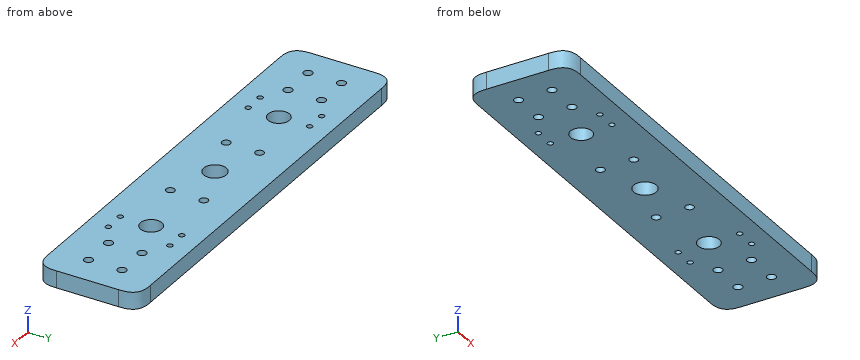
from build123d import *

# Parameters (mm, degrees)
SKETCH1_W                     = 320
SKETCH1_H                     = 76.2
BOSS_EXTRUDE1_DEPTH           = 12.7
M6_CLEARANCE_HOLE1_D          = 6.6
FILLET1_SIZE                  = 15
TAP_DRILL_FOR_M5X0_8_TAP1_D   = 4.2
SKETCH8_R                     = 8
CUT_EXTRUDE1_DEPTH            = 165.963329386
M6_CLEARANCE_HOLE2_D          = 6.4
M16_CLEARANCE_HOLE1_OUTLINE_R = 8.5
M16_CLEARANCE_HOLE1_DEPTH     = 12.7


with BuildPart() as part:
    # Sketch1 → Boss-Extrude1 (new body)
    with BuildSketch(Plane.XY):
        Rectangle(SKETCH1_W, SKETCH1_H)
    extrude(amount=BOSS_EXTRUDE1_DEPTH)

    # M6 Clearance Hole1 (through all)
    with Locations(Plane(origin=(0, 0, 0), x_dir=(-1, 0, 0), z_dir=(0, 0, -1))):
        with Locations((137.5, -12.5), (112.5, -12.5), (112.5, 12.5), (137.5, 12.5), (-112.5, -12.5), (-137.5, -12.5), (-112.5, 12.5), (-137.5, 12.5)):
            Hole(M6_CLEARANCE_HOLE1_D / 2)

    # Fillet1
    # a fillet whose section is not a circle: 15 mm, written as the material it takes off along each edge
    with BuildSketch(Plane(origin=(-160, 38.1, -37.5), x_dir=(1, 0, 0), z_dir=(0, 0, 1)), Plane(origin=(-160, -38.1, -37.5), x_dir=(0, 1, 0), z_dir=(0, 0, 1))) as fillet1_piece_1:
        with BuildLine():
            add(Edge.make_bspline([(FILLET1_SIZE, 0), (FILLET1_SIZE * 0.831801948466, 0), (FILLET1_SIZE * 0.663603896932, 0), (FILLET1_SIZE * 0.292893218813, -FILLET1_SIZE * 0.0716919198361), (FILLET1_SIZE * 0.0716919198361, -FILLET1_SIZE * 0.292893218813), (0, -FILLET1_SIZE * 0.663603896932), (0, -FILLET1_SIZE * 0.831801948466), (0, -FILLET1_SIZE)], knots=[0, 0, 0, 0, 0, 0, 0.5, 0.5, 1, 1, 1, 1, 1, 1], degree=5))
            Line((0, -FILLET1_SIZE), (0, 0))
            Line((0, 0), (FILLET1_SIZE, 0))
        make_face()
    extrude(amount=87.7, mode=Mode.SUBTRACT)
    with BuildSketch(Plane(origin=(160, 38.1, -37.5), x_dir=(-1, 0, 0), z_dir=(0, 0, 1)), Plane(origin=(160, -38.1, -37.5), x_dir=(0, 1, 0), z_dir=(0, 0, 1))) as fillet1_piece_2:
        with BuildLine():
            add(Edge.make_bspline([(FILLET1_SIZE, 0), (FILLET1_SIZE * 0.831801948466, 0), (FILLET1_SIZE * 0.663603896932, 0), (FILLET1_SIZE * 0.292893218813, FILLET1_SIZE * 0.0716919198361), (FILLET1_SIZE * 0.0716919198361, FILLET1_SIZE * 0.292893218813), (0, FILLET1_SIZE * 0.663603896932), (0, FILLET1_SIZE * 0.831801948466), (0, FILLET1_SIZE)], knots=[0, 0, 0, 0, 0, 0, 0.5, 0.5, 1, 1, 1, 1, 1, 1], degree=5))
            Line((0, FILLET1_SIZE), (0, 0))
            Line((0, 0), (FILLET1_SIZE, 0))
        make_face()
    extrude(amount=87.7, mode=Mode.SUBTRACT)

    # Tap Drill for M5x0.8 Tap1 (through all)
    with Locations(Plane.XY.offset(12.7)):
        with Locations((-95.121488027, -23), (-80.121488027, -23), (-95.121488027, 23), (-80.121488027, 23), (80.121488027, -23), (95.121488027, -23), (95.121488027, 23), (80.121488027, 23)):
            Hole(TAP_DRILL_FOR_M5X0_8_TAP1_D / 2)

    # Sketch8 → Cut-Extrude1 (cut, through all)
    with BuildSketch(Plane.XY.offset(12.7)):
        with Locations((-80, 0)):
            Circle(SKETCH8_R)
        with Locations((80, 0)):
            Circle(SKETCH8_R)
    extrude(amount=-CUT_EXTRUDE1_DEPTH, mode=Mode.SUBTRACT)

    # M6 Clearance Hole2 (through all)
    with Locations(Plane.XY.offset(12.7)):
        with Locations((-35, -12.5), (-35, 12.5), (35, 12.5), (35, -12.5)):
            Hole(M6_CLEARANCE_HOLE2_D / 2)

    # M16 Clearance Hole1: read off the stored shape, not the designer's step
    # M16 Clearance Hole1 outline → M16 Clearance Hole1 (cut)
    with BuildSketch(Plane.XY):
        Circle(M16_CLEARANCE_HOLE1_OUTLINE_R)
    extrude(amount=M16_CLEARANCE_HOLE1_DEPTH, mode=Mode.SUBTRACT)


solid = part.part
Read the model definition and answer for the solid it produces. Units are mm, in the model's axes. Round coordinates to 2 decimals unless told otherwise and drop trailing zeros. Loops run counter-clockwise (first coordinate to the right, second up) from the corner with the lowest first, then second, coordinate; pieces in that order, holes last. Notation, with made-up numbers: (2.5, -6.5) - (15.5, -6.5) arc R21 ccw to (15.5, 31.5) - close; hole circle Ø10 at (17.25, -4.75). An arc over 180 degrees is marked (long way). One line per question, with ' | ' between items. Start each with the question number.
Q1. Section C-C on x = 3 is taken. Give the vertices of the cut face in (y, z), plus the area to 3 significant figures.
Q2. Find the intervals of material crossed by L1, parallel to Y at x = 35, z = 10; L2, parallel to Y at x = 37.5, z = 8.25; L3, parallel to X at y = -6.5, z = 9.5, in increasing order.
Q3. Section B-B on y = 12.5 is taken. Give the vertices of the cut face in (x, z), plus the area to 3 significant figures.
Q4. Section A-A on x = 112.5 is taken. Give the vertices of the cut face in (y, z).
Q5. A flat-ended cylindrical pin translates along its axis: pin 1 (3.5 mm diameter, centred on x = 95.12, y = 23, fed in from +Z). Find the tip coordinate at first contact, or state that the pin passes through.
Q6. Section D-D on z = 5.5 is taken. Count the separate pieces of the cut face and the enclosed holes in it, plus the area to 3 significant figures.
Established:
1) outline: (-38.1, 0) - (-7.95, 0) - (-7.95, 12.7) - (-38.1, 12.7) - close; (7.95, 0) - (38.1, 0) - (38.1, 12.7) - (7.95, 12.7) - close | area: 766 mm²
2) L1: -38.1 to -15.7, -9.3 to 9.3, 15.7 to 38.1 | L2: -38.1 to -14.5, -10.5 to 10.5, 14.5 to 38.1 | L3: -160 to -84.66, -75.34 to -5.48, 5.48 to 75.34, 84.66 to 160
3) outline: (-160, 0) - (-140.8, 0) - (-140.8, 12.7) - (-160, 12.7) - close; (-134.2, 0) - (-115.8, 0) - (-115.8, 12.7) - (-134.2, 12.7) - close; (-109.2, 0) - (-38.2, 0) - (-38.2, 12.7) - (-109.2, 12.7) - close; (-31.8, 0) - (31.8, 0) - (31.8, 12.7) - (-31.8, 12.7) - close; (38.2, 0) - (109.2, 0) - (109.2, 12.7) - (38.2, 12.7) - close; (115.8, 0) - (134.2, 0) - (134.2, 12.7) - (115.8, 12.7) - close; (140.8, 0) - (160, 0) - (160, 12.7) - (140.8, 12.7) - close | area: 3,570 mm²
4) outline: (-38.1, 0) - (-15.8, 0) - (-15.8, 12.7) - (-38.1, 12.7) - close; (-9.2, 0) - (9.2, 0) - (9.2, 12.7) - (-9.2, 12.7) - close; (15.8, 0) - (38.1, 0) - (38.1, 12.7) - (15.8, 12.7) - close
5) pin 1: through
6) separate pieces: 1 | enclosed holes: 23 | area: 23,100 mm²
